Part model, mm, in its own coordinate system. A direction names the side the tool comes from. Round coordinates to 2 decimals unless told otherwise and drop trailing zeros. Loops run counter-clockwise (first coordinate to the right, second up) from the corner with the lowest first, then second, coordinate; pieces in that order, holes last.
from build123d import *

# Parameters (mm, degrees)
F0_R     = 4.445
F0_R_2   = 17.907
F1_DEPTH = 6.35


with BuildPart() as f1:
    # F0 (on Top) → F1 (new body)
    with BuildSketch(Plane.XY):
        with BuildLine():
            Line((40.391009, 11.792125), (27.161882, 11.792125))
            ThreePointArc((27.161882, 11.792125), (22.671754, 13.651997), (20.811882, 18.142125))
            Line((20.811882, 18.142125), (20.811882, 31.058542))
            ThreePointArc((20.811882, 31.058542), (17.092138, 40.038798), (8.111882, 43.758542))
            Line((8.111882, 43.758542), (5.682427, 43.758542))
            ThreePointArc((5.682427, 43.758542), (-3.297829, 40.038798), (-7.017573, 31.058542))
            Line((-7.017573, 31.058542), (-7.017573, 17.829415))
            ThreePointArc((-7.017573, 17.829415), (-8.877445, 13.339287), (-13.367573, 11.479415))
            Line((-13.367573, 11.479415), (-26.283991, 11.479415))
            ThreePointArc((-26.283991, 11.479415), (-35.264247, 7.759671), (-38.983991, -1.220585))
            Line((-38.983991, -1.220585), (-38.983991, -3.65004))
            ThreePointArc((-38.983991, -3.65004), (-35.264247, -12.630296), (-26.283991, -16.35004))
            Line((-26.283991, -16.35004), (-13.054863, -16.35004))
            ThreePointArc((-13.054863, -16.35004), (-8.564735, -18.209912), (-6.704863, -22.70004))
            Line((-6.704863, -22.70004), (-6.704863, -35.616458))
            ThreePointArc((-6.704863, -35.616458), (-2.985119, -44.596714), (5.995137, -48.316458))
            Line((5.995137, -48.316458), (8.424592, -48.316458))
            ThreePointArc((8.424592, -48.316458), (17.404848, -44.596714), (21.124592, -35.616458))
            Line((21.124592, -35.616458), (21.124592, -22.38733))
            ThreePointArc((21.124592, -22.38733), (22.984464, -17.897202), (27.474592, -16.03733))
            Line((27.474592, -16.03733), (40.391009, -16.03733))
            ThreePointArc((40.391009, -16.03733), (49.371265, -12.317586), (53.091009, -3.33733))
            Line((53.091009, -3.33733), (53.091009, -0.907875))
            ThreePointArc((53.091009, -0.907875), (49.371265, 8.072381), (40.391009, 11.792125))
        make_face()
        with Locations((6.882834, -38.473555)):
            Circle(F0_R, mode=Mode.SUBTRACT)
        with Locations((43.248107, -2.449633)):
            Circle(F0_R, mode=Mode.SUBTRACT)
        with Locations((-29.141088, -2.108283)):
            Circle(F0_R, mode=Mode.SUBTRACT)
        with Locations((7.053509, -2.278958)):
            Circle(F0_R_2, mode=Mode.SUBTRACT)
        with Locations((7.224184, 33.91564)):
            Circle(F0_R, mode=Mode.SUBTRACT)
    extrude(amount=F1_DEPTH)


solid = f1.part
1) Tool access for faces 4 (the face through (34, 11.792, 3)), 5 (the face through (7, -48.316, 3)), 6 (the face through (-6.705, -29, 3)): list every direction of +Z, -Z, +X, -X, +Y, -Y with a clear straight run to the whole face (end or side of a thin tool).
Values:
face 4: +Z, -Z, +X, +Y
face 5: +Z, -Z, +X, -X, -Y
face 6: +Z, -Z, -X, -Y
2) Slice it at C-C, the plane z = 2.25. Give the number of separate pieces and of enclosed holes in the cut face, then the cut area to 3 significant figures.
Values:
separate pieces: 1
enclosed holes: 5
area: 2,850 mm2
3) Slice it at A-A, the plane x = 45.5. Give the cut face in (y, z), then the cut area to 3 significant figures.
Values:
outline: (-14.96, 0) - (-6.28, 0) - (-6.28, 6.35) - (-14.96, 6.35) - close; (1.38, 0) - (10.72, 0) - (10.72, 6.35) - (1.38, 6.35) - close
area: 114 mm2
4) Slice it at D-D, the plane x = -18.5. Give the cut face in (y, z).
Values:
outline: (-16.35, 0) - (11.48, 0) - (11.48, 6.35) - (-16.35, 6.35) - close
5) Slice it at B-B, the plane y = 5. Give the cut face in (x, z), then the cut area to 3 significant figures.
Values:
outline: (-37.36, 0) - (-9.31, 0) - (-9.31, 6.35) - (-37.36, 6.35) - close; (23.41, 0) - (51.63, 0) - (51.63, 6.35) - (23.41, 6.35) - close
area: 357 mm2
6) Drop flat-ended pins along their axis: pin 1 Ø5.5 at (x, y) = (7.22, 33.92) entering from -Z; pin 2 Ø3 at (x, z) = (-19.5, 3) entering from +Y; pin 3 Ø1.9 at (x, z) = (36.5, 3) entering from -Y; pin 4 Ø1.9 at (y, z) = (21, 3) entering from -X. Give the stop position or say it passes through.
Values:
pin 1: passes through
pin 2: stops at y = 11.48
pin 3: stops at y = -16.04
pin 4: stops at x = -7.02
7) Mould opens along X. For faces 1 (the face through (47.488, -1.114, 3.131)), 2 (the face through (-38.984, -2, 3)), 3 (the face through (-20, -16.35, 3)) say: released by +X, released by -X, zero draft, split by the parting line, or undercut.
Values:
face 1: undercut
face 2: released by -X
face 3: zero draft
8) Wall check: line 1 along X through (y, z) = (-1.5, 1.5); line 2 along Y through (x, z) = (-22, 2); line 3 along Y through (x, z) = (35.5, 2.5). Give the ranges that are in metal, low to high.
Values:
line 1: x = -38.98 to -33.54, -24.74 to -10.84, 24.94 to 38.91, 47.59 to 53.09
line 2: y = -16.35 to 11.48
line 3: y = -16.04 to 11.79
